from build123d import *

# Parameters (mm, degrees)
SKETCH1_R             = 6.5
SKETCH1_R_2           = 2
BOSS_EXTRUDE1_DEPTH   = 5
CHAMFER1_SIZE         = 0.5
CHAMFER1_SIZE2        = 0.243866294
CHAMFER1_PART_2_SIZE  = 0.5
CHAMFER1_PART_2_SIZE2 = 0.243866294


with BuildPart() as part:
    # Sketch1 → Boss-Extrude1 (new body)
    with BuildSketch(Plane.XY):
        Circle(SKETCH1_R)
        Circle(SKETCH1_R_2, mode=Mode.SUBTRACT)
    extrude(amount=BOSS_EXTRUDE1_DEPTH)

    # Chamfer1
    chamfer1_edges = [part.edges().sort_by_distance(p)[0] for p in [
        (-6.5, 0, 0),
    ]]
    chamfer1_side = [part.faces().sort_by_distance(p)[0] for p in [
        (-6.316152237, 0, 0),
    ]]
    chamfer(chamfer1_edges, length=CHAMFER1_SIZE, length2=CHAMFER1_SIZE2, reference=chamfer1_side[0])

    # Chamfer1 part 2
    chamfer1_part_2_edges = [part.edges().sort_by_distance(p)[0] for p in [
        (-6.5, 0, 5),
    ]]
    chamfer1_part_2_side = [part.faces().sort_by_distance(p)[0] for p in [
        (-6.5, 0, 2.5),
    ]]
    chamfer(chamfer1_part_2_edges, length=CHAMFER1_PART_2_SIZE, length2=CHAMFER1_PART_2_SIZE2, reference=chamfer1_part_2_side[0])


solid = part.part
Here's how the part is built. I have some questions about the finished solid (model axes, mm). Coordinates: 2 decimals unless noted, no trailing zeros. Loops run counter-clockwise (first coordinate to the right, second up) from the corner with the lowest first, then second, coordinate; pieces in that order, holes last. Notation, with made-up numbers: (-15, 2) -> (-9, 2) arc R15 cw to (-9, 19) -> close; hole circle Ø8 at (76, -2.75). An arc over 180 degrees is marked (long way). Use one line per item in the form item = value. Start each with the question number.
(1) Please list where these lines run through material, in increasing order: line 1 along Y through (x, z) = (0, 3); line 2 along X through (y, z) = (1.5, 3.15); line 3 along X through (y, z) = (1, 1).
(2) If we section it at A-A (x = 0): Please give me the cut outline in (y, z), then the cut area to 3 significant figures.
(3) We'd pull the mould along Y, two halves only. Please class faces 1 (the face through (0, -2, 2)), 2 (the face through (-5.158, -3.955, 2.342)), 3 (the face through (3, 0, 0)): pulls with the +Y half, pulls with the -Y half, needs draft (parallel to the pull), parting line crosses it, or undercut.
(4) Will these pins go through, and if not, where does the flat tip stop? pin 1 (2 mm diameter, centred on x = -4, z = 4.5, fed in from +Y); pin 2 (1.5 mm diameter, centred on x = 2.5, z = 1.5, fed in from -Y); pin 3 (2 mm diameter, centred on y = 4, z = 2.5, fed in from +X).
(5) If we section it at C-C (z = 2.1): Please give me the cut outline in (x, y).
Verdict:
q1.line_1 = -6.5 to -2, 2 to 6.5
q1.line_2 = -6.32 to -1.32, 1.32 to 6.32
q1.line_3 = -6.42 to -1.73, 1.73 to 6.42
q2.outline = (-6.5, 0.24) -> (-6, 0) -> (-2, 0) -> (-2, 5) -> (-6.26, 5) -> (-6.5, 4.5) -> close; (2, 0) -> (6, 0) -> (6.5, 0.24) -> (6.5, 4.5) -> (6.26, 5) -> (2, 5) -> close
q2.area = 44.8 mm²
q3.face_1 = undercut
q3.face_2 = parting line crosses it
q3.face_3 = needs draft
q4.pin_1 = 5.77
q4.pin_2 = -6.26
q4.pin_3 = 5.77
q5.outline = circle Ø13 at (0, 0); hole circle Ø4 at (0, 0)
